Design review of the part shown in the three views and the two pictorial views. Dimensions are in mm from the part's minimum x, y and z. A direction names the side the tool comes from. Round coordinates to 2 decimals unless told otherwise and drop trailing zeros. Write each loop counter-clockwise with the first axis right and the second up, starting at its lowest first coordinate (ties: lowest second). Pieces come first, ordered by that corner, then holes. Notation, with made-up numbers: (17, 50.25) -> (76, 50.25) arc R23 cw to (76, 61.25) -> close; hole circle Ø5 at (14.25, -29). An arc over 180 degrees is marked (long way). One line per question, with ' | ' between items. Start each with the question number.
1) Insertion check: pin 1 Ø10 at (x, y) = (10.5, 16.5) entering from -Z; pin 2 Ø22.5 at (x, z) = (21.5, 41) entering from -Y; pin 3 Ø5.5 at (x, y) = (18, 62.5) entering from +Z; pin 4 Ø8 at (x, z) = (24.5, 30.5) entering from +Y. Each pin has a flat end and moves straight along its axis. Give the tip position at first contact, or say it passes through.
2) Consider section C-C (x = 25). Give the boundary of the cut face in (y, z).
3) Consider section D-D (y = 32.5). Give the boundary of the cut face in (x, z), then the cut area to 3 significant figures.
4) Mouldability with a two-part tool opening along Y and no side actions: class the marked faces 1, 2 and 3 as +Y half, -Y half, draft (parallel to the pull), parting line (faces both ways), or undercut.
5) For probe 1 along Y at (x, z) = (26, 17.5); probe 2 along Y at (x, z) = (13.5, 46); probe 3 along Z at (x, y) = (11.5, 34), list the stretches that pass through material, from the lowest coordinate up.
6) Consider section A-A (z = 12). Give the boundary of the cut face in (x, y), then the cut area to 4 significant figures.
7) For the marked faces 4, 5 and 6, list the 3-axis set-ups (+Z, -Z, +X, -X, +Y, -Y) from which the entire face can be reached by the end or side of a thin tool; tool diameter is ignored.
8) Consider section B-B (z = 42). Give the boundary of the cut face in (x, y).
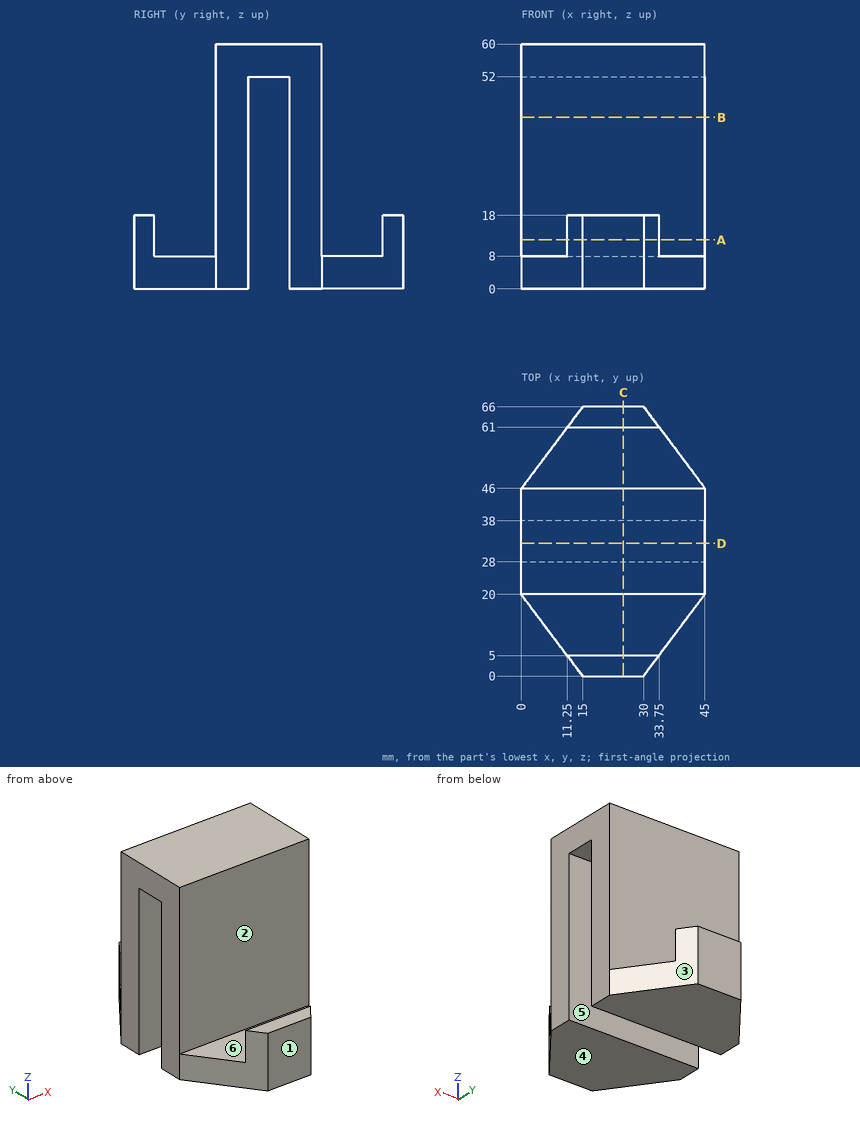
From the geometry:
1) pin 1: stops at z = 0 | pin 2: stops at y = 20 | pin 3: stops at z = 18 | pin 4: stops at y = 46
2) outline: (0, 0) -> (28, 0) -> (28, 52) -> (38, 52) -> (38, 0) -> (66, 0) -> (66, 18) -> (61, 18) -> (61, 8) -> (46, 8) -> (46, 60) -> (20, 60) -> (20, 8) -> (5, 8) -> (5, 18) -> (0, 18) -> close
3) outline: (0, 52) -> (45, 52) -> (45, 60) -> (0, 60) -> close | area: 360 mm2
4) face 1: -Y half | face 2: undercut | face 3: +Y half
5) probe 1: y = 0 to 5, 20 to 28, 38 to 46, 61 to 66 | probe 2: y = 20 to 28, 38 to 46 | probe 3: z = 52 to 60
6) outline: (0, 20) -> (45, 20) -> (45, 28) -> (0, 28) -> close; (0, 38) -> (45, 38) -> (45, 46) -> (0, 46) -> close; (11.25, 5) -> (15, 0) -> (30, 0) -> (33.75, 5) -> close; (11.25, 61) -> (33.75, 61) -> (30, 66) -> (15, 66) -> close | area: 907.5 mm2
7) face 4: -Z, +X, -X, +Y, -Y | face 5: -Z, +X, -X | face 6: +Z, +X, -X
8) outline: (0, 20) -> (45, 20) -> (45, 28) -> (0, 28) -> close; (0, 38) -> (45, 38) -> (45, 46) -> (0, 46) -> close
